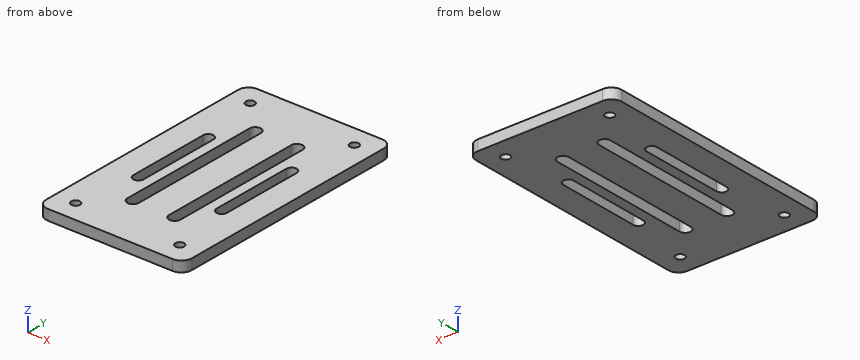
Autodesk Inventor part; units mm, degrees
ref_plane "YZ Plane" through (0, 0, 0) normal (1, 0, 0) x (0, 1, 0)
ref_plane "XZ Plane" through (0, 0, 0) normal (0, 1, 0) x (-1, 0, 0)
ref_plane "XY Plane" through (0, 0, 0) normal (0, 0, 1) x (1, 0, 0)
sketch "Skizze1" plane through (0, 0, 0) normal (0, 0, 1) x (1, 0, 0)
  line L0 (5, 0) -> (65, 0)
  line L1 (70, 5) -> (70, 115)
  line L2 (65, 120) -> (5, 120)
  line L3 (0, 115) -> (0, 5)
  arc A0 (70, 115) -> (65, 120) centre (65, 115) ccw
  arc A1 (65, 0) -> (70, 5) centre (65, 5) ccw
  arc A2 (0, 5) -> (5, 0) centre (5, 5) ccw
  arc A3 (5, 120) -> (0, 115) centre (5, 115) ccw
  point P0 (0, 0)
  point P1 (70, 120)
  point P2 (70, 0)
  dimension "d0" = 120
  dimension "d1" = 70
  dimension "d3" = 5
extrude "Extrusion1" add sketch "Skizze1" along normal blind 5
sketch "Skizze2" plane through (0, 0, 5) normal (0, 0, 1) x (1, 0, 0)
  circle A0 centre (60, 10) radius 2.1
  circle A1 centre (10, 10) radius 2.1
  circle A2 centre (10, 110) radius 2.1
  circle A3 centre (60, 110) radius 2.1
  point P0 (0, 0)
  dimension "d6" = 4.2
  dimension "d7" = 4.2
  dimension "d8" = 4.2
  dimension "d9" = 4.2
  dimension "d10" = 100
  dimension "d11" = 50
  dimension "d12" = 10
  dimension "d13" = 10
extrude "Extrusion2" cut sketch "Skizze2" against normal through all
sketch "Skizze3" plane through (0, 0, 5) normal (0, 0, 1) x (1, 0, 0)
  line L0 (15, 80) -> (15, 40) construction
  line L1 (12.5, 80) -> (12.5, 40)
  line L2 (17.5, 40) -> (17.5, 80)
  arc A0 (17.5, 80) -> (12.5, 80) centre (15, 80) ccw
  arc A1 (12.5, 40) -> (17.5, 40) centre (15, 40) ccw
  line L3 (65, 120) -> (5, 120)
  line L4 (35, 120) -> (35, 0) construction
  line L5 (0, 115) -> (0, 5)
  line L6 (0, 60) -> (70, 60) construction
  line L7 (70, 5) -> (70, 115)
  line L8 (55, 80) -> (55, 40) construction
  line L9 (57.5, 80) -> (57.5, 40)
  line L10 (52.5, 40) -> (52.5, 80)
  arc A2 (57.5, 80) -> (52.5, 80) centre (55, 80) ccw
  arc A3 (52.5, 40) -> (57.5, 40) centre (55, 40) ccw
  point P0 (0, 0)
  point P1 (15, 60)
  point P2 (55, 60)
  dimension "d16" = 40
  dimension "d18" = 2.5
  dimension "d20" = 20
  dimension "d21" = 0
extrude "Extrusion3" cut sketch "Skizze3" against normal through all
sketch "Skizze4" plane through (0, 0, 5) normal (0, 0, 1) x (1, 0, 0)
  line L0 (45, 25) -> (45, 95) construction
  line L1 (47.75, 25) -> (47.75, 95)
  line L2 (42.25, 95) -> (42.25, 25)
  arc A0 (42.25, 25) -> (47.75, 25) centre (45, 25) ccw
  arc A1 (47.75, 95) -> (42.25, 95) centre (45, 95) ccw
  line L3 (5, 0) -> (65, 0)
  line L4 (35, 0) -> (35, 120) construction
  line L5 (65, 120) -> (5, 120)
  line L6 (70, 5) -> (70, 115)
  line L7 (70, 60) -> (0, 60) construction
  line L8 (0, 115) -> (0, 5)
  line L9 (25, 25) -> (25, 95) construction
  line L10 (22.25, 25) -> (22.25, 95)
  line L11 (27.75, 95) -> (27.75, 25)
  arc A2 (22.25, 25) -> (27.75, 25) centre (25, 25) ccw
  arc A3 (27.75, 95) -> (22.25, 95) centre (25, 95) ccw
  arc A4 (17.5, 80) -> (12.5, 80) centre (15, 80) ccw
  arc A5 (12.5, 40) -> (17.5, 40) centre (15, 40) ccw
  point P0 (0, 0)
  point P1 (45, 60)
  point P2 (25, 60)
  point P3 (25, 60)
  point P4 (35, 60)
  dimension "d24" = 2.75
  dimension "d28" = 10
  dimension "d35" = 15
extrude "Extrusion4" cut sketch "Skizze4" against normal up to surface (5 mm away)
properties part number "103.009.01_Grundplatte_Stopper" material "PMMA-Kunststoff"
CAD build for the part. Positions are in the model's coordinates, mm. Coordinates: 2 decimals unless noted, no trailing zeros. Write each loop counter-clockwise with the first axis right and the second up, starting at its lowest first coordinate (ties: lowest second). Pieces come first, ordered by that corner, then holes.
(1) Cut at A-A, the plane y = 46. List the corners of the cut face in (x, z).
(2) Drill centre lines: probe 1 along Y at (x, z) = (60, 1.95); probe 2 along X at (y, z) = (88, 0.9); probe 3 along X at (y, z) = (48.5, 3). Where is each one in solid material? Low to high.
(3) Cut at C-C, the plane y = 10. List the corners of the cut face in (x, z).
(4) Flat gauge pins, fed straight in: pin 1 (2.5 mm diameter, centred on y = 56.5, z = 2, fed in from -X); pin 2 (2.5 mm diameter, centred on x = 10, y = 110, fed in from -Z). Where does each tip first touch, or does it go through?
(5) Cut at B-B, the plane x = 55. List the corners of the cut face in (y, z).
(6) Cut at D-D, the plane x = 10. List the corners of the cut face in (y, z).
Geometry says:
1. outline: (0, 0) - (12.5, 0) - (12.5, 5) - (0, 5) - close; (17.5, 0) - (22.25, 0) - (22.25, 5) - (17.5, 5) - close; (27.75, 0) - (42.25, 0) - (42.25, 5) - (27.75, 5) - close; (47.75, 0) - (52.5, 0) - (52.5, 5) - (47.75, 5) - close; (57.5, 0) - (70, 0) - (70, 5) - (57.5, 5) - close
2. probe 1: y = 0 to 7.9, 12.1 to 107.9, 112.1 to 120
2. probe 2: x = 0 to 22.25, 27.75 to 42.25, 47.75 to 70
2. probe 3: x = 0 to 12.5, 17.5 to 22.25, 27.75 to 42.25, 47.75 to 52.5, 57.5 to 70
3. outline: (0, 0) - (7.9, 0) - (7.9, 5) - (0, 5) - close; (12.1, 0) - (57.9, 0) - (57.9, 5) - (12.1, 5) - close; (62.1, 0) - (70, 0) - (70, 5) - (62.1, 5) - close
4. pin 1: stops at x = 0
4. pin 2: passes through
5. outline: (0, 0) - (37.5, 0) - (37.5, 5) - (0, 5) - close; (82.5, 0) - (120, 0) - (120, 5) - (82.5, 5) - close
6. outline: (0, 0) - (7.9, 0) - (7.9, 5) - (0, 5) - close; (12.1, 0) - (107.9, 0) - (107.9, 5) - (12.1, 5) - close; (112.1, 0) - (120, 0) - (120, 5) - (112.1, 5) - close
